Here's how the part is built. I have some questions about the finished solid (model axes, mm). Face numbers are marked on the shaded views. A direction names the side the tool comes from. Coordinates: 2 decimals unless noted, no trailing zeros. Write each loop counter-clockwise with the first axis right and the second up, starting at its lowest first coordinate (ties: lowest second). Pieces come first, ordered by that corner, then holes.
Item 1: If I drill on line 1 (X direction, y = 0, z = -16.45) (3 decimals); line 2 (Y direction, x = 0, z = 22), over which ranges is the centre line in solid material (lowest first)?
Item 2: I'm going to push flat-ended pins straight in: pin 1 Ø10 at (x, y) = (-32.33, -32.33) entering from +Z; pin 2 Ø5 at (x, z) = (19, 13) entering from +Y; pin 3 Ø10 at (y, z) = (-16, -7) entering from +X. Where does each tip first touch, or does it pass through?
Item 3: For the marked faces 1 and 2, which set-ups out of +Z, -Z, +X, -X, +Y, -Y let a thin tool reach every point of the face, with its end or its side?
Item 4: If we section it at A-A (y = 0): Please give me the cut outline in (x, z) (3 decimals).
Item 5: We'd pull the mould along X, two halves only. Please class the marked faces 3, 4 and 5: +X half, -X half, draft (parallel to the pull), parting line (faces both ways), or undercut.
Item 6: If we section it at B-B (x = 45.72): Please give me the cut outline in (y, z) (3 decimals), then the cut area to 3 significant figures.
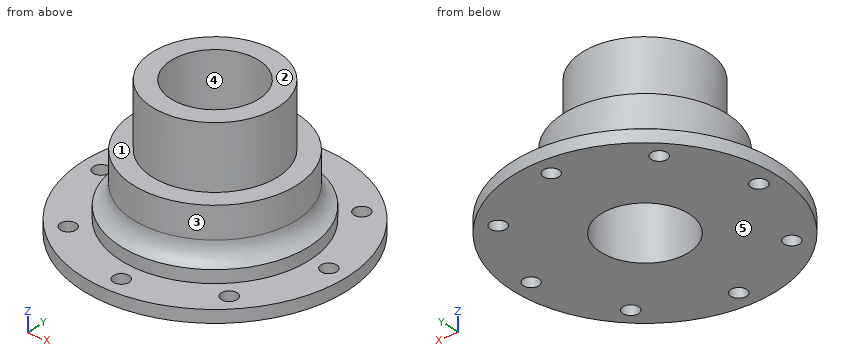
Autodesk Fusion 360 part; units mm, degrees
sketch "Sketch1" plane through (0, 0, 0) normal (0, 1, 0) x (1, 0, 0)
  line L0 (25.4, -38.1) -> (25.4, -12.7)
  line L1 (25.4, -12.7) -> (33.02, -12.7)
  line L2 (33.02, -12.7) -> (33.02, 0)
  arc A0 (38.1, 7.62) -> (33.02, 0) centre (41.275, 0) ccw
  line L3 (38.1, 7.62) -> (38.1, 12.7)
  line L4 (25.4, -38.1) -> (0, -38.1)
  line L5 (38.1, 12.7) -> (53.34, 12.7)
  line L6 (53.34, 12.7) -> (53.34, 17.78)
  line L7 (53.34, 17.78) -> (0, 17.78)
  line L8 (0, -38.1) -> (0, 17.78)
revolve "Revolve1" add sketch "Sketch1" angle 360 about axis through (0, 0, 38.1) along (0, 0, -1)
sketch "Sketch2" plane through (0, 0, -12.7) normal (0, 0, 1) x (-1, 0, 0)
  circle A0 centre (0, 0) radius 53.34
  circle A1 centre (0, 0) radius 38.1
  circle A2 centre (0, -45.72) radius 3.175
  dimension "d2" = 6.35
extrude "Extrude1" cut sketch "Sketch2" against normal up to surface (5.08 mm away) contours A2
pattern_circular "C-Pattern1" count 8 over 360 about axis through (0, 0, 1.75) along (0, 0, 1) of "Extrude1"
sketch "Sketch3" plane through (0, 0, 38.1) normal (0, 0, 1) x (-1, 0, 0)
  circle A0 centre (0, 0) radius 25.4
  circle A1 centre (0, 0) radius 17.78
extrude "Extrude2" cut sketch "Sketch3" against normal up to surface (55.88 mm away) contours A1
Answer list:
1. line 1: x = -53.34 to -48.895, -42.545 to -17.78, 17.78 to 42.545, 48.895 to 53.34
1. line 2: y = -25.4 to -17.78, 17.78 to 25.4
2. pin 1: stops at z = -12.7
2. pin 2: stops at y = 28.59
2. pin 3: stops at x = 36.47
3. face 1: +Z
3. face 2: +Z, +X, -X, +Y, -Y
4. outline: (-53.34, -17.78) - (-48.895, -17.78) - (-48.895, -12.7) - (-53.34, -12.7) - close; (-42.545, -17.78) - (-17.78, -17.78) - (-17.78, 38.1) - (-25.4, 38.1) - (-25.4, 12.7) - (-33.02, 12.7) - (-33.02, 0) arc R8.255 cw to (-38.1, -7.62) - (-38.1, -12.7) - (-42.545, -12.7) - close; (17.78, -17.78) - (42.545, -17.78) - (42.545, -12.7) - (38.1, -12.7) - (38.1, -7.62) arc R8.255 cw to (33.02, 0) - (33.02, 12.7) - (25.4, 12.7) - (25.4, 38.1) - (17.78, 38.1) - close; (48.895, -17.78) - (53.34, -17.78) - (53.34, -12.7) - (48.895, -12.7) - close
5. face 3: parting line
5. face 4: undercut
5. face 5: draft
6. outline: (-27.474, -17.78) - (-3.175, -17.78) - (-3.175, -12.7) - (-27.474, -12.7) - close; (3.175, -17.78) - (27.474, -17.78) - (27.474, -12.7) - (3.175, -12.7) - close
6. area: 247 mm2
